Autodesk Inventor part; units mm, degrees
ref_plane "작업 평면1" through (0, 0, 8.3) normal (0, 0, 1) x (1, 0, 0)
ref_plane "YZ Plane" through (0, 0, 0) normal (1, 0, 0) x (0, 1, 0)
ref_plane "XZ Plane" through (0, 0, 0) normal (0, 1, 0) x (-1, 0, 0)
sketch "스케치1" plane through (0, 0, 0) normal (1, 0, 0) x (0, 1, 0)
  circle A0 centre (0, 0) radius 5.3
  circle A1 centre (0, 0) radius 5
  line L0 (4, 3) -> (-4, 3)
  circle A2 centre (0, 0) radius 8.3
  line L1 (4, 3) -> (11.6093, 3)
  line L2 (-4, 3) -> (-10.334, 3)
  line L3 (11.6093, -38.4) -> (-10.334, -38.4) construction
  circle A3 centre (0, -76.8) radius 5.3
  circle A4 centre (0, -76.8) radius 5
  line L4 (4, -79.8) -> (-4, -79.8)
  circle A5 centre (0, -76.8) radius 8.3
  line L5 (4, -79.8) -> (11.6093, -79.8)
  line L6 (-4, -79.8) -> (-10.334, -79.8)
  line L7 (-8.3, 0) -> (-8.3, -76.8)
  line L8 (-5.3, 0) -> (-5.3, -76.8)
  line L9 (0, -8.3) -> (-5.3, -8.3)
  line L10 (0, -68.5) -> (-5.3, -68.5)
  point P0 (0, 3)
  point P1 (0, -79.8)
  point P2 (-4.3692, -79.8)
  point P3 (4.3692, -79.8)
  point P4 (7.7389, 3)
  point P5 (4.3692, 3)
  point P6 (-4.3692, 3)
  point P7 (-7.7389, 3)
  point P8 (-7.7389, -79.8)
  point P9 (7.7389, -79.8)
  dimension "d0" = 10.6
  dimension "d1" = 3
  dimension "d2" = 10
  dimension "d3" = 16.6
  dimension "d4" = 38.4
extrude "돌출1" add sketch "스케치1" along normal blind 20 contours L8 A2 L2 A0 | A0 L1 A2 L8 | L8 A5 L7 A2 | A2 L9 L8 | A5 L8 A3 L6 | L10 A5 L8 | A5 L5 A3 L8
ref_plane "작업 평면1" through (0, 0, 8.3) normal (0, 0, 1) x (1, 0, 0)
sketch "스케치3" plane through (0, -8.3, -76.8) normal (0, -1, 0) x (1, 0, 0)
  line L0 (0, 76.8) -> (0, 0)
  line L1 (0, 0) -> (20, 0)
  line L2 (20, 76.8) -> (20, 0)
  line L3 (0, 76.8) -> (20, 76.8)
  line L4 (0, 0) -> (0, -3)
  line L5 (0, -3) -> (20, -3)
  line L6 (20, 0) -> (20, -3)
  line L7 (0, 0) -> (20, 0)
  line L8 (0, 79.8) -> (0, 76.8)
  line L9 (0, 76.8) -> (20, 76.8)
  line L10 (20, 79.8) -> (20, 76.8)
  line L11 (0, 79.8) -> (20, 79.8)
  line L12 (20, 38.4) -> (0, 38.4) construction
  line L13 (0, 79.8) -> (20, 79.8)
  line L14 (10, 79.8) -> (10, -3) construction
  circle A0 centre (10, 19.2) radius 2.5
  line L15 (6, 12.3) -> (14, 12.3)
  line L16 (14, 12.3) -> (14, 4.3)
  line L17 (14, 4.3) -> (6, 4.3)
  line L18 (6, 4.3) -> (6, 12.3)
  line L19 (0, 8.3) -> (20, 8.3)
  line L20 (6, 12.3) -> (14, 4.3) construction
  line L21 (14, 12.3) -> (6, 4.3) construction
  circle A1 centre (10, 57.6) radius 2.5
  line L22 (6, 64.5) -> (14, 64.5)
  line L23 (14, 64.5) -> (14, 72.5)
  line L24 (14, 72.5) -> (6, 72.5)
  line L25 (6, 72.5) -> (6, 64.5)
  line L26 (0, 68.5) -> (20, 68.5)
  line L27 (6, 64.5) -> (14, 72.5) construction
  line L28 (14, 64.5) -> (6, 72.5) construction
  circle A2 centre (10, 0) radius 1.25
  circle A3 centre (10, 76.8) radius 1.25
  point P0 (10, 8.3)
  point P1 (10, 68.5)
  dimension "d10" = 38.4
  dimension "d11" = 10
  dimension "d12" = 5
  dimension "d13" = 19.2
  dimension "d14" = 8
  dimension "d15" = 8
  dimension "d20" = 2.5
extrude "돌출3" cut sketch "스케치3" against normal blind 20 contours A3 L3 | L3 A3 | A2 L1 | L1 A2 | A0 | A1
extrude "돌출4" add sketch "스케치3" along normal blind 2 contours L26 L23 L22 L25 | L25 L24 L23 L26 | L19 L16 L17 L18 | L18 L15 L16 L19
properties part number "pipe_holder_typeB"
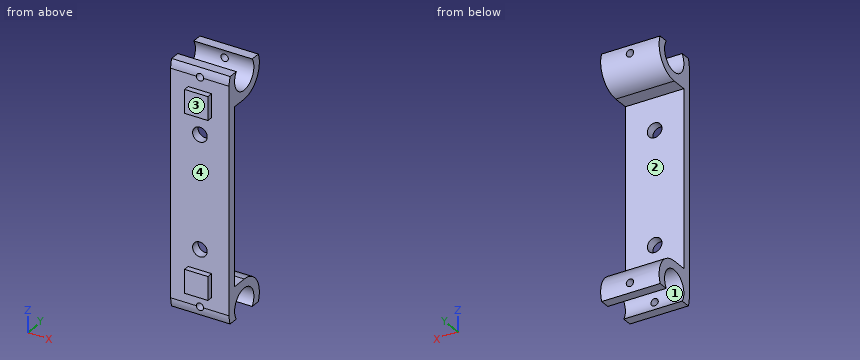
Model file for the job. Use its own axes, mm. Face numbers are marked on the shaded views. A direction names the side the tool comes from. Round coordinates to 2 decimals unless told otherwise and drop trailing zeros. Order: outer loops, then holes, each group sorted by start corner. A loop starts at its lowest first (then second) coordinate and runs counter-clockwise, first axis right, second up.
(1) Pin check, flat tips, straight feed: pin 1 (9.5 mm diameter, centred on y = 0, z = 0, fed in from -X); pin 2 (0.6 mm diameter, centred on y = -9, z = -70, fed in from +X); pin 3 (6.5 mm diameter, centred on x = 10, z = -19.2, fed in from +Y); pin 4 (1 mm diameter, centred on x = 9.5, y = -9.5, fed in from +Z). Stop position of each tip, or through.
(2) Pull direction Z, two halves, no side cores. Call the marked faces 3 and 4: released by +Z, released by -Z, zero draft, split by the parting line, or undercut.
(3) Band-saw the part on C-C (x = 16.75). List the corners of the cut face in (y, z), then the cut area to 3 significant figures.
(4) 3-axis set-ups, long thin cutter, end or side, ignore diameter. For the marked faces 1 and 2: which of +Z, -Z, +X, -X, +Y, -Y reach the whole face in a straight line?
(5) Band-saw the part on A-A (z = -19.2). List the corners of the cut face in (x, y), then the cut area to 3 significant figures.
(6) Band-saw the part on B-B (y = 3). List the corners of the cut face in (x, z).
(7) Band-saw the part on D-D (x = 10). Give the number of separate pieces and of enclosed holes in the cut face, then the cut area to 3 significant figures.
(8) Drill centre lines: line 1 (Z direction, x = 10, y = -7.1); line 2 (X direction, y = -6.8, z = -76.8); line 3 (Z direction, x = 6.75, y = 0). Where is each one in solid material? Low to high.
Verdict:
1. pin 1: passes through
1. pin 2: stops at x = 14
1. pin 3: stops at y = -5.3
1. pin 4: stops at z = -4.3
2. face 3: zero draft
2. face 4: undercut
3. outline: (-8.3, -76.8) arc R8.3 ccw to (-7.74, -79.8) - (-4.37, -79.8) arc R5.3 cw (long way) to (4.37, -79.8) - (7.74, -79.8) arc R8.3 ccw to (0, -68.5) - (-5.3, -68.5) - (-5.3, -8.3) - (0, -8.3) arc R8.3 ccw to (7.74, 3) - (4.37, 3) arc R5.3 cw (long way) to (-4.37, 3) - (-7.74, 3) arc R8.3 ccw to (-8.3, 0) - close
3. area: 376 mm2
4. face 1: +X, -X
4. face 2: +X, -X, +Y
5. outline: (0, -8.3) - (7.5, -8.3) - (7.5, -5.3) - (0, -5.3) - close; (12.5, -8.3) - (20, -8.3) - (20, -5.3) - (12.5, -5.3) - close
5. area: 45.0 mm2
6. outline: (0, -72.43) - (20, -72.43) - (20, -69.06) - (0, -69.06) - close; (0, -7.74) - (20, -7.74) - (20, -4.37) - (0, -4.37) - close
7. separate pieces: 7
7. enclosed holes: 0
7. area: 347 mm2
8. line 1: z = -79.8 to -78.05, -75.55 to -60.1, -55.1 to -21.7, -16.7 to -1.25, 1.25 to 3
8. line 2: x = 0 to 8.75, 11.25 to 20
8. line 3: z = -71.5 to -68.5, -8.3 to -5.3
